Print and shaded views of the part. All mm, measured from the part's lowest x, y and z. A direction names the side the tool comes from. Round coordinates to 2 decimals unless told otherwise and drop trailing zeros. Write each loop counter-clockwise with the first axis right and the second up, starting at its lowest first coordinate (ties: lowest second). Pieces come first, ordered by that corner, then holes. Notation, with made-up numbers: (35.25, -31.5) -> (92.25, -31.5) arc R14 ccw to (92.25, -24.5) -> close; hole circle Ø5 at (0.25, 47). An arc over 180 degrees is marked (long way). Return JSON: item names as keys, results as strings. Group by question number.
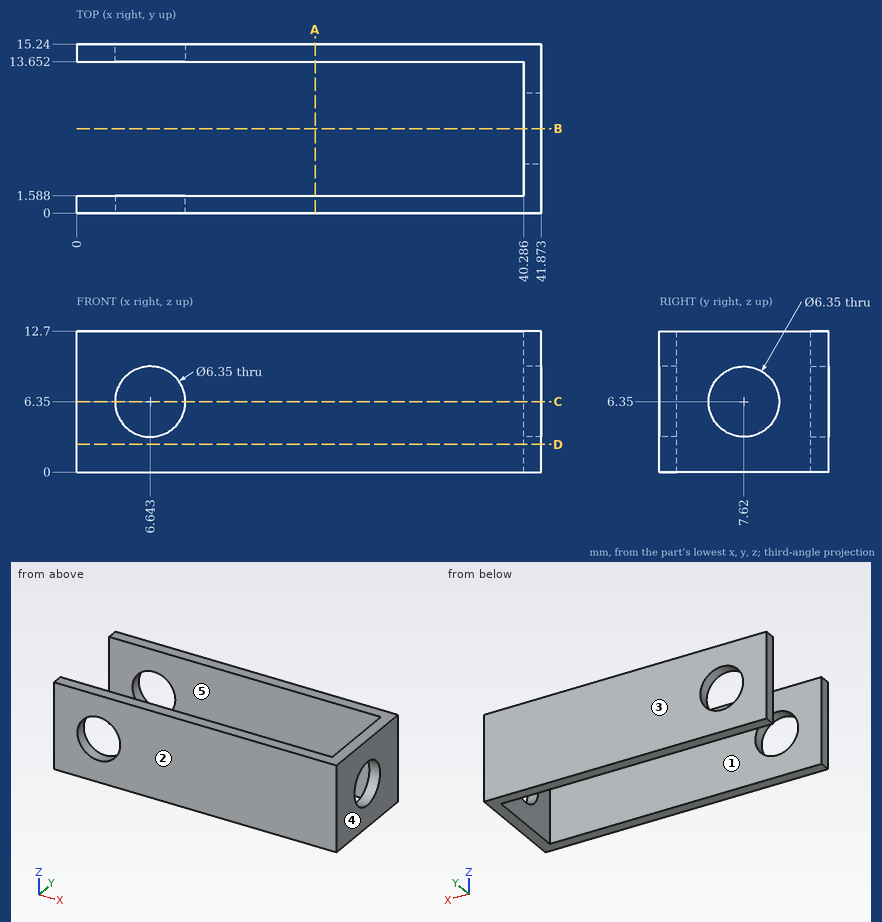
Item 1: Which spindle directions (+Z, -Z, +X, -X, +Y, -Y) get a long thin tool onto all of the face, cutting with end or side? Do the marked faces 4 and 5. Say none if no direction does.
Item 2: Cut at C-C (z = 6.35). Write the cut outline in (x, y) (1 decimal).
Item 3: Wall check: L1, parallel to Z at x = 41.2, y = 7.62 (1 decimal); L2, parallel to Y at x = 21, z = 10; L3, parallel to X at y = 5, z = 10.5 (1 decimal). Give the ranges that are in metal, low to high.
Item 4: Cut at A-A (x = 21.5). Write the cut outline in (y, z).
Item 5: Two-plate mould, pull along Y, no slides. Class the marked faces 1, 2 and 3: released by +Y, released by -Y, zero draft, split by the parting line, or undercut.
Item 6: Cut at D-D (z = 2.5). Write the cut outline in (x, y) (1 decimal), then the cut area to 3 significant figures.
Item 7: Flat gauge pins, fed straight in: P1, Ø6, axis at y = 12, z = 3, coming from the -X side; P2, Ø1, axis at y = 2.5, z = 1.5, coming from the -X side. Where does each tip first touch, or does it go through?
Item 8: Cut at B-B (y = 7.62). Write the cut outline in (x, z) (1 decimal).
Checks:
{
 "1": {"face 4": "+Z, -Z, +X, +Y, -Y", "face 5": "+Z, -Z, -X"},
 "2": {"outline": "(0, 0) -> (3.5, 0) -> (3.5, 1.6) -> (0, 1.6) -> close; (0, 13.7) -> (3.5, 13.7) -> (3.5, 15.2) -> (0, 15.2) -> close; (9.8, 0) -> (41.9, 0) -> (41.9, 4.4) -> (40.3, 4.4) -> (40.3, 1.6) -> (9.8, 1.6) -> close; (9.8, 13.7) -> (40.3, 13.7) -> (40.3, 10.8) -> (41.9, 10.8) -> (41.9, 15.2) -> (9.8, 15.2) -> close"},
 "3": {"L1": "z = 0 to 3.2, 9.5 to 12.7", "L2": "y = 0 to 1.59, 13.65 to 15.24", "L3": "x = 40.3 to 41.9"},
 "4": {"outline": "(0, 0) -> (1.59, 0) -> (1.59, 12.7) -> (0, 12.7) -> close; (13.65, 0) -> (15.24, 0) -> (15.24, 12.7) -> (13.65, 12.7) -> close"},
 "5": {"face 1": "undercut", "face 2": "released by -Y", "face 3": "released by +Y"},
 "6": {"outline": "(0, 0) -> (41.9, 0) -> (41.9, 15.2) -> (0, 15.2) -> (0, 13.7) -> (40.3, 13.7) -> (40.3, 1.6) -> (0, 1.6) -> close", "area": "152 mm2"},
 "7": {"P1": "stops at x = 0", "P2": "stops at x = 40.29"},
 "8": {"outline": "(40.3, 0) -> (41.9, 0) -> (41.9, 3.2) -> (40.3, 3.2) -> close; (40.3, 9.5) -> (41.9, 9.5) -> (41.9, 12.7) -> (40.3, 12.7) -> close"}
}
